from build123d import *

# Parameters (mm, degrees)
CROQUIS1_W              = 32
CROQUIS1_H              = 45
SALIENTE_EXTRUIR1_DEPTH = 5
CROQUIS2_W              = 16
CROQUIS2_H              = 10
SALIENTE_EXTRUIR2_DEPTH = 5
CROQUIS3_R              = 1.5
CORTAR_EXTRUIR1_DEPTH   = 33.20636583
CROQUIS4_W              = 10
CROQUIS4_H              = 16
SALIENTE_EXTRUIR3_DEPTH = 5
CROQUIS5_R              = 1.5
CORTAR_EXTRUIR2_DEPTH   = 35.960692213
CROQUIS6_W              = 10
CROQUIS6_H              = 45
SALIENTE_EXTRUIR4_DEPTH = 5


with BuildPart() as part:
    # Croquis1 → Saliente-Extruir1 (new body)
    with BuildSketch(Plane(origin=(0, 0, 0), x_dir=(1, 0, 0), z_dir=(0, 1, 0))):
        Rectangle(CROQUIS1_W, CROQUIS1_H)
    extrude(amount=SALIENTE_EXTRUIR1_DEPTH)

    # Croquis2 → Saliente-Extruir2 (add, through all)
    with BuildSketch(Plane(origin=(0, 5, 0), x_dir=(1, 0, 0), z_dir=(0, 1, 0))):
        with Locations((0, 22.5)):
            Rectangle(CROQUIS2_W, CROQUIS2_H)
    saliente_extruir2 = extrude(amount=-SALIENTE_EXTRUIR2_DEPTH)

    # Croquis3 → Cortar-Extruir1 (cut, through all)
    with BuildSketch(Plane(origin=(0, 5, 0), x_dir=(1, 0, 0), z_dir=(0, 1, 0))):
        with Locations(Location((0, 24.5, 0), (0, 0, 270))):
            Circle(CROQUIS3_R)
    cortar_extruir1 = extrude(amount=-CORTAR_EXTRUIR1_DEPTH, mode=Mode.SUBTRACT)

    # Simetría1: Saliente-Extruir2, Cortar-Extruir1 across plane
    add(saliente_extruir2.mirror(Plane.XY))
    add(cortar_extruir1.mirror(Plane.XY), mode=Mode.SUBTRACT)

    # Croquis4 → Saliente-Extruir3 (add, through all)
    with BuildSketch(Plane(origin=(0, 5, 0), x_dir=(1, 0, 0), z_dir=(0, 1, 0))):
        with Locations((-16, 0)):
            Rectangle(CROQUIS4_W, CROQUIS4_H)
    extrude(amount=-SALIENTE_EXTRUIR3_DEPTH)

    # Croquis5 → Cortar-Extruir2 (cut, through all)
    with BuildSketch(Plane(origin=(0, 5, 0), x_dir=(1, 0, 0), z_dir=(0, 1, 0))):
        with Locations(Location((-18, 0, 0), (0, 0, 270))):
            Circle(CROQUIS5_R)
    extrude(amount=-CORTAR_EXTRUIR2_DEPTH, mode=Mode.SUBTRACT)

    # Croquis6 → Saliente-Extruir4 (add)
    with BuildSketch(Plane(origin=(0, 5, 0), x_dir=(1, 0, 0), z_dir=(0, 1, 0))):
        with Locations((21, 0)):
            Rectangle(CROQUIS6_W, CROQUIS6_H)
    extrude(amount=-SALIENTE_EXTRUIR4_DEPTH)


solid = part.part
Can you work these out from the model? Positions are in its coordinate system, mm. A direction names the side the tool comes from. Round coordinates to 2 decimals unless told otherwise and drop trailing zeros. Loops run counter-clockwise (first coordinate to the right, second up) from the corner with the lowest first, then second, coordinate; pieces in that order, holes last. Notation, with made-up numbers: (76.25, 55.5) - (114.25, 55.5) arc R24 cw to (114.25, 72.5) - close; hole circle Ø11 at (-36.75, -8.5). An arc over 180 degrees is marked (long way). Answer in a Markdown table with one row per item. Add a question column.
Q1. I want a section at D-D on x = 0. List the corners of the cut face in (y, z) for me, and give its area (3 significant figures).
Q2. For pin 1 Ø2.5 at (x, y) = (14, 3.5) entering from -Z; pin 2 Ø1.5 at (y, z) = (2, -15) entering from -X; pin 3 Ø1.5 at (y, z) = (3.5, -25.5) entering from -X, each with a flat end and sliding along its axis, tell me the tip position at first contact or that it passes through.
Q3. Which directions (+Z, -Z, +X, -X, +Y, -Y) give clear straight access to the entire face, cutting with the end or side of a thin tool? Please do faces 4 (the flat face through (-12, 2, -22.5)), 5 (the flat face through (8, 3, 25)), 6 (the flat face through (-16, 2, 15)).
Q4. I want a section at B-B on x = -18. List the corners of the cut face in (y, z) for me, and give its area (3 significant figures).
Q5. We'd pull the mould along X, two halves only. Please class faces 1 (the cylindrical face through (-16.735, 2.535, 0.806)), 2 (the flat face through (-21, 3, 0)), 3 (the flat face through (-12, 2, 22.5)): pulls with the +X half, pulls with the -X half, needs draft (parallel to the pull), parting line crosses it, or undercut.
Q6. I want a section at C-C on y = 4.3. List the corners of the cut face in (x, z) for me, and give its area (3 significant figures).
Q7. I need wall thicknesses on L1, parallel to X at y = 2.05, z = 0; L2, parallel to X at y = 1.35, z = -8.5; L3, parallel to X at y = 3.45, z = 24.5. Which ranges of each line are inside material? Lowest first, please.
Q8. I want a section at A-A on z = 24.5. List the corners of the cut face in (x, y) for me, and give its area (3 significant figures).
A:
| question | item | result |
|---|---|---|
| 1 | outline | (0, -27.5) - (5, -27.5) - (5, -26) - (0, -26) - close; (0, -23) - (5, -23) - (5, 23) - (0, 23) - close; (0, 26) - (5, 26) - (5, 27.5) - (0, 27.5) - close |
| 1 | area | 245 mm^2 |
| 2 | pin 1 | z = -22.5 |
| 2 | pin 2 | x = -16 |
| 2 | pin 3 | x = -8 |
| 3 | face 4 | -Z, -X, +Y, -Y |
| 3 | face 5 | +Z, +X, +Y, -Y |
| 3 | face 6 | +Z, -X, +Y, -Y |
| 4 | outline | (0, -8) - (5, -8) - (5, -1.5) - (0, -1.5) - close; (0, 1.5) - (5, 1.5) - (5, 8) - (0, 8) - close |
| 4 | area | 65.0 mm^2 |
| 5 | face 1 | undercut |
| 5 | face 2 | pulls with the -X half |
| 5 | face 3 | needs draft |
| 6 | outline | (-21, -8) - (-16, -8) - (-16, -22.5) - (-8, -22.5) - (-8, -27.5) - (8, -27.5) - (8, -22.5) - (26, -22.5) - (26, 22.5) - (8, 22.5) - (8, 27.5) - (-8, 27.5) - (-8, 22.5) - (-16, 22.5) - (-16, 8) - (-21, 8) - close; hole circle Ø3 at (-18, 0); hole circle Ø3 at (0, -24.5); hole circle Ø3 at (0, 24.5) |
| 6 | area | 2,110 mm^2 |
| 7 | L1 | -21 to -19.5, -16.5 to 26 |
| 7 | L2 | -16 to 26 |
| 7 | L3 | -8 to -1.5, 1.5 to 8 |
| 8 | outline | (-8, 0) - (-1.5, 0) - (-1.5, 5) - (-8, 5) - close; (1.5, 0) - (8, 0) - (8, 5) - (1.5, 5) - close |
| 8 | area | 65.0 mm^2 |
